CAD build for the part. Positions are in the model's coordinates, mm. A direction names the side the tool comes from. Round coordinates to 2 decimals unless told otherwise and drop trailing zeros. Loops run counter-clockwise (first coordinate to the right, second up) from the corner with the lowest first, then second, coordinate; pieces in that order, holes last. Notation, with made-up numbers: M 1.25,25 L 21.25,25 A4 cw 21.25,31 Z; hole C 24,88 d9. An arc over 180 degrees is marked long. Use a Markdown table: item, result. Add a question column.
(1) Band-saw the part on B-B, the plane y = 7. Write the cut outline in (x, z).
(2) Two-plate mould, pull along X, no slides. Class faces 1 (the face through (54, 13.9, 23.5)), 2 (the face through (52, 26.6, 22)), 3 (the face through (63.51, 0.81, -31.11)), 4 (the face through (-61.49, 0.81, 28.89)): released by +X, released by -X, zero draft, split by the parting line, or undercut.
(3) Band-saw the part on A-A, the plane x = -62.5. Write the cut outline in (y, z).
(4) Which spindle directions (+Z, -Z, +X, -X, +Y, -Y) get a long thin tool onto all of the face, cutting with end or side? Do faces 5 (the face through (-8, 9, 13)), 6 (the face through (-8, 9, -13)), 7 (the face through (-46, 9, 0)). Say none if no direction does.
(5) Wall check: L1, parallel to X at y = 0.75, z = 30; L2, parallel to Y at x = 15.5, z = 25; L3, parallel to Y at x = -6.5, z = -9. Give the ranges that are in metal, low to high.
(6) Band-saw the part on D-D, the plane x = 27. Write the cut outline in (y, z), and give its area (3 significant figures).
(7) Flat gauge pins, fed straight in: P1, Ø13, axis at x = -26.5, z = -6, coming from the +Y side; P2, Ø2, axis at x = -49, z = -26, coming from the +Y side; P3, Ø4, axis at x = 10.5, y = 7.5, coming from the -Z side. Where does each tip first touch, or does it go through?
(8) Band-saw the part on C-C, the plane z = -30. Write the cut outline in (x, y).
from build123d import *

# Parameters (mm, degrees)
SKETCH1_W           = 135
SKETCH1_H           = 70
BOSS_EXTRUDE1_DEPTH = 1.6
CUT_EXTRUDE1_REACH  = 78.051
SKETCH2_R           = 1.5
SKETCH3_R           = 2.5
BOSS_EXTRUDE2_DEPTH = 25
SKETCH4_W           = 77
SKETCH4_H           = 26
BOSS_EXTRUDE3_DEPTH = 14


with BuildPart() as part:
    # Sketch1 → Boss-Extrude1 (new body)
    with BuildSketch(Plane(origin=(0, 0, 0), x_dir=(1, 0, 0), z_dir=(0, 1, 0))):
        Rectangle(SKETCH1_W, SKETCH1_H)
    extrude(amount=BOSS_EXTRUDE1_DEPTH)

    # Sketch2 → Cut-Extrude1 (cut, up to next)
    with BuildSketch(Plane(origin=(0, 1.6, 0), x_dir=(1, 0, 0), z_dir=(0, 1, 0)), mode=Mode.PRIVATE) as cut_extrude1_sk1:
        with Locations(Location((62.5, 30, 0), (0, 0, 270))):
            Circle(SKETCH2_R)
    cut_extrude1_tool1 = extrude(cut_extrude1_sk1.sketch, amount=-CUT_EXTRUDE1_REACH, mode=Mode.PRIVATE) & part.part
    # Sketch2 → Cut-Extrude1 (cut, up to next)
    with BuildSketch(Plane(origin=(0, 1.6, 0), x_dir=(1, 0, 0), z_dir=(0, 1, 0)), mode=Mode.PRIVATE) as cut_extrude1_sk2:
        with Locations(Location((-62.5, 30, 0), (0, 0, 270))):
            Circle(SKETCH2_R)
    cut_extrude1_tool2 = extrude(cut_extrude1_sk2.sketch, amount=-CUT_EXTRUDE1_REACH, mode=Mode.PRIVATE) & part.part
    # Sketch2 → Cut-Extrude1 (cut, up to next)
    with BuildSketch(Plane(origin=(0, 1.6, 0), x_dir=(1, 0, 0), z_dir=(0, 1, 0)), mode=Mode.PRIVATE) as cut_extrude1_sk3:
        with Locations(Location((-62.5, -30, 0), (0, 0, 270))):
            Circle(SKETCH2_R)
    cut_extrude1_tool3 = extrude(cut_extrude1_sk3.sketch, amount=-CUT_EXTRUDE1_REACH, mode=Mode.PRIVATE) & part.part
    # Sketch2 → Cut-Extrude1 (cut, up to next)
    with BuildSketch(Plane(origin=(0, 1.6, 0), x_dir=(1, 0, 0), z_dir=(0, 1, 0)), mode=Mode.PRIVATE) as cut_extrude1_sk4:
        with Locations(Location((62.5, -30, 0), (0, 0, 270))):
            Circle(SKETCH2_R)
    cut_extrude1_tool4 = extrude(cut_extrude1_sk4.sketch, amount=-CUT_EXTRUDE1_REACH, mode=Mode.PRIVATE) & part.part
    add(cut_extrude1_tool1.solids().sort_by_distance((62.5, 1.6, -30))[0], mode=Mode.SUBTRACT)
    add(cut_extrude1_tool2.solids().sort_by_distance((-62.5, 1.6, -30))[0], mode=Mode.SUBTRACT)
    add(cut_extrude1_tool3.solids().sort_by_distance((-62.5, 1.6, 30))[0], mode=Mode.SUBTRACT)
    add(cut_extrude1_tool4.solids().sort_by_distance((62.5, 1.6, 30))[0], mode=Mode.SUBTRACT)

    # Sketch3 → Boss-Extrude2 (add)
    with BuildSketch(Plane(origin=(0, 1.6, 0), x_dir=(1, 0, 0), z_dir=(0, 1, 0))):
        with Locations(Location((52.5, -21.5, 0), (0, 0, 90))):
            Circle(SKETCH3_R)
    extrude(amount=BOSS_EXTRUDE2_DEPTH)

    # Sketch4 → Boss-Extrude3 (add)
    with BuildSketch(Plane(origin=(0, 1.6, 0), x_dir=(1, 0, 0), z_dir=(0, 1, 0))):
        with Locations((-7.5, 0)):
            Rectangle(SKETCH4_W, SKETCH4_H)
    extrude(amount=BOSS_EXTRUDE3_DEPTH)


solid = part.part
Return value:
| question | item | result |
|---|---|---|
| 1 | outline | M -46,-13 L 31,-13 L 31,13 L -46,13 Z; C 52.5,21.5 d5 |
| 2 | face 1 | split by the parting line |
| 2 | face 2 | zero draft |
| 2 | face 3 | undercut |
| 2 | face 4 | undercut |
| 3 | outline | M 0,-35 L 1.6,-35 L 1.6,-31.5 L 0,-31.5 Z; M 0,-28.5 L 1.6,-28.5 L 1.6,28.5 L 0,28.5 Z; M 0,31.5 L 1.6,31.5 L 1.6,35 L 0,35 Z |
| 4 | face 5 | +Z, +X, -X, +Y |
| 4 | face 6 | -Z, +X, -X, +Y |
| 4 | face 7 | +Z, -Z, -X, +Y |
| 5 | L1 | -67.5 to -64, -61 to 61, 64 to 67.5 |
| 5 | L2 | 0 to 1.6 |
| 5 | L3 | 0 to 15.6 |
| 6 | outline | M 0,-35 L 1.6,-35 L 1.6,-13 L 15.6,-13 L 15.6,13 L 1.6,13 L 1.6,35 L 0,35 Z |
| 6 | area | 476 mm^2 |
| 7 | P1 | y = 15.6 |
| 7 | P2 | y = 1.6 |
| 7 | P3 | z = -13 |
| 8 | outline | M -67.5,0 L -64,0 L -64,1.6 L -67.5,1.6 Z; M -61,0 L 61,0 L 61,1.6 L -61,1.6 Z; M 64,0 L 67.5,0 L 67.5,1.6 L 64,1.6 Z |
